Geometry check sheet. Reference: drawing and pictorial views, mm from the part's lowest x, y, z. A direction names the side the tool comes from. Round coordinates to 2 decimals unless told otherwise and drop trailing zeros. Order: outer loops, then holes, each group sorted by start corner. A loop starts at its lowest first (then second) coordinate and runs counter-clockwise, first axis right, second up. Notation, with made-up numbers: (-5.75, 39) -> (3.25, 39) arc R21 cw to (3.25, 67) -> close; hole circle Ø10 at (-34.75, 77). An arc over 180 degrees is marked (long way). Put each result on its own line as item: value.
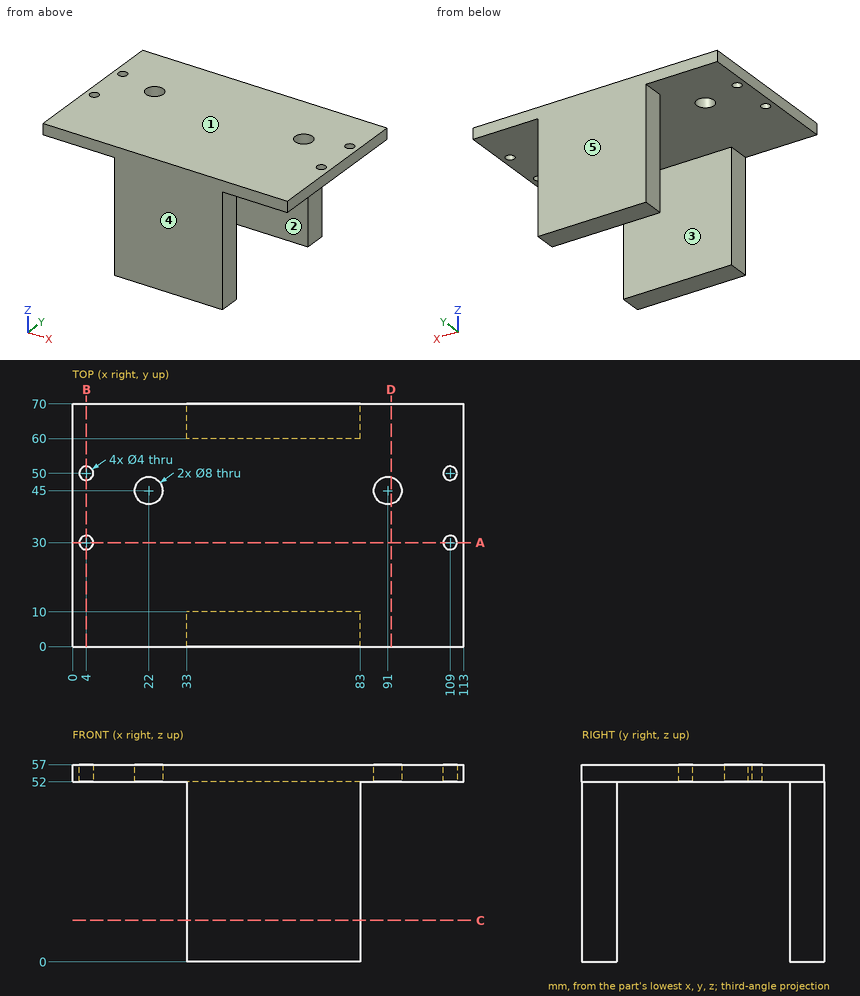
Item 1: Sectioned sample at C-C, the plane z = 12. Record the boundary of the cut face in (x, y), then the cut area to 3 significant figures.
Geometry check:
outline: (33, 0) -> (83, 0) -> (83, 10) -> (33, 10) -> close; (33, 60) -> (83, 60) -> (83, 70) -> (33, 70) -> close
area: 1,000 mm2
Item 2: Sectioned sample at B-B, the plane x = 4. Record the boundary of the cut face in (y, z), then the cut area to 3 significant figures.
Geometry check:
outline: (0, 52) -> (28, 52) -> (28, 57) -> (0, 57) -> close; (32, 52) -> (48, 52) -> (48, 57) -> (32, 57) -> close; (52, 52) -> (70, 52) -> (70, 57) -> (52, 57) -> close
area: 310 mm2
Item 3: Material ranges on line 1 along Y through (x, z) = (109, 56); line 2 along Y through (x, z) = (61, 40); line 3 along Y through (x, z) = (22, 53.7), recorded low to high.
Geometry check:
line 1: 0 to 28, 32 to 48, 52 to 70
line 2: 0 to 10, 60 to 70
line 3: 0 to 41, 49 to 70
Item 4: Release check for a two-part mould opening along Y. For the marked faces 3, 4 and 5 record: pulls with the +Y half, pulls with the -Y half, needs draft (parallel to the pull), parting line crosses it, or undercut.
Geometry check:
face 3: undercut
face 4: pulls with the -Y half
face 5: pulls with the +Y half
Item 5: Tool access check on the marked faces 1 and 2. Record the directions out of +Z, -Z, +X, -X, +Y, -Y that give a thin tool (end or side, any length) a straight path to the whole face; none if there is none.
Geometry check:
face 1: +Z, +X, -X, +Y, -Y
face 2: -Z, +X, -X
Item 6: Sectioned sample at A-A, the plane y = 30. Record the boundary of the cut face in (x, z), then the cut area to 3 significant figures.
Geometry check:
outline: (0, 52) -> (2, 52) -> (2, 57) -> (0, 57) -> close; (6, 52) -> (107, 52) -> (107, 57) -> (6, 57) -> close; (111, 52) -> (113, 52) -> (113, 57) -> (111, 57) -> close
area: 525 mm2
Item 7: Sectioned sample at D-D, the plane x = 92. Record the boundary of the cut face in (y, z), then the cut area to 3 significant figures.
Geometry check:
outline: (0, 52) -> (41.13, 52) -> (41.13, 57) -> (0, 57) -> close; (48.87, 52) -> (70, 52) -> (70, 57) -> (48.87, 57) -> close
area: 311 mm2
Item 8: Depth check by flat-ended pin: pin 1 Ø7 at (x, y) = (91, 45) entering from +Z; pin 2 Ø11 at (y, z) = (67.5, 36) entering from +X; pin 3 Ø21 at (x, y) = (62, 30.5) entering from -Z; pin 4 Ø3 at (y, z) = (63, 23.5) entering from -X. Enter the tip coordinate at first touch or a pass-through.
Geometry check:
pin 1: through
pin 2: x = 83
pin 3: z = 52
pin 4: x = 33
